from build123d import *

# Parameters (mm, degrees)
F1_DEPTH = 8
F2_R     = 20
F3_R     = 5


with BuildPart() as f1:
    # F0 (on Front) → F1 (new body)
    with BuildSketch(Plane.XZ):
        Polygon((250, 0), (0, 300), (0, 0), align=None)
        Polygon((30, 30), (30, 217.138502), (185.948752, 30), align=None, mode=Mode.SUBTRACT)
    extrude(amount=F1_DEPTH)

    # F2
    f2_edges = [f1.edges().sort_by_distance(p)[0] for p in [
        (30, -4, 30),
        (185.948752, -4, 30),
        (30, -4, 217.138502),
    ]]
    fillet(f2_edges, radius=F2_R)

    # F3
    f3_edges = [f1.edges().sort_by_distance(p)[0] for p in [
        (250, -4, 0),
        (0, -4, 300),
        (0, -4, 0),
    ]]
    fillet(f3_edges, radius=F3_R)


solid = f1.part
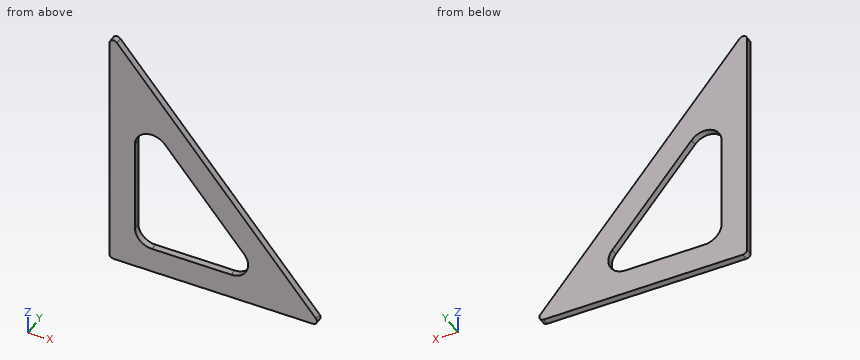
Source: CAD feature listing. Evaluate the final solid. Frame: model axes, mm. Round coordinates to 2 decimals unless told otherwise and drop trailing zeros. Loops run counter-clockwise (first coordinate to the right, second up) from the corner with the lowest first, then second, coordinate; pieces in that order, holes last. Notation, with made-up numbers: (-34, -29.75) - (-25, -29.75) arc R22 cw to (-25, -3.75) - close; hole circle Ø7 at (-33.75, 86). An arc over 180 degrees is marked (long way). Write item = value, one per line. Start each with the question number.
Item 1: Section query B-B on z = 165.5. Output: boundary loops of the cut face in (x, y).
Item 2: Material intervals for line 1 (X direction, y = -6.25, z = 114); line 2 (Z direction, x = 89.5, y = -3); line 3 (X direction, y = -0.5, z = 37), sorted ascending.
Item 3: Section query C-C on x = 90.5. Output: boundary loops of the cut face in (y, z), plus the area to 3 significant figures.
Item 4: First-contact query: pin 1 Ø1 at (y, z) = (-3.5, 236) entering from +X; pin 2 Ø1 at (y, z) = (-5.5, 86.5) entering from +X; pin 3 Ø2.5 at (x, y) = (99.5, -3.5) entering from +Z. Flat tips, straight axial feed; report the tip coordinate or a pass-through.
Item 5: Section query A-A on y = -1.5. Output: boundary loops of the cut face in (x, z), plus the area to 3 significant figures.
Item 6: Section query D-D on x = 228. Output: boundary loops of the cut face in (y, z).
Results list:
q1.outline = (0, -8) - (30.33, -8) - (30.33, 0) - (0, 0) - close; (73.03, -8) - (112.08, -8) - (112.08, 0) - (73.03, 0) - close
q2.line_1 = 0 to 30, 115.95 to 155
q2.line_2 = 0 to 30, 145.74 to 192.6
q2.line_3 = 0 to 34.8, 158.45 to 219.17
q3.outline = (-8, 0) - (0, 0) - (0, 30) - (-8, 30) - close; (-8, 144.54) - (0, 144.54) - (0, 191.4) - (-8, 191.4) - close
q3.area = 615 mm²
q4.pin_1 = 53.75
q4.pin_2 = 178.33
q4.pin_3 = 182.1
q5.outline = (0, 5) arc R5 ccw to (5, 0) - (239.32, 0) arc R5 ccw to (243.17, 8.2) - (8.84, 289.39) arc R5 ccw to (0, 286.19) - close; hole (30, 50) arc R20 ccw to (50, 30) - (143.25, 30) arc R20 ccw to (158.61, 62.8) - (65.36, 174.7) arc R20 ccw to (30, 161.9) - close
q5.area = 23,900 mm²
q6.outline = (-8, 0) - (0, 0) - (0, 26.4) - (-8, 26.4) - close
